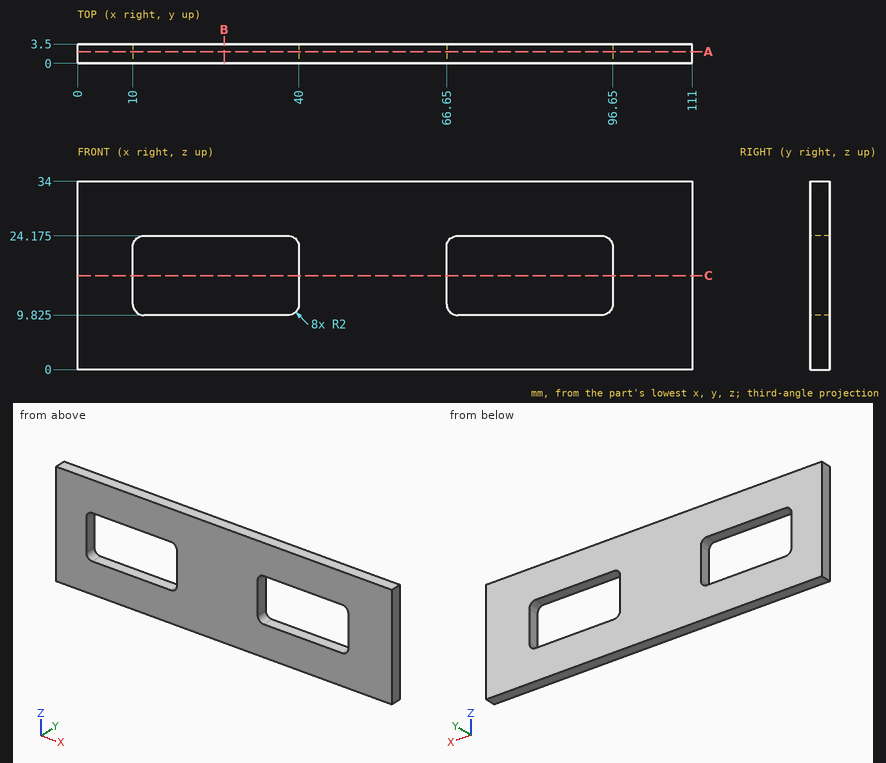
Design review of the part shown in the three views and the two pictorial views. Dimensions are in mm from the part's minimum x, y and z. Coordinates: 2 decimals unless noted, no trailing zeros. Loops run counter-clockwise (first coordinate to the right, second up) from the corner with the lowest first, then second, coordinate; pieces in that order, holes last. Notation, with made-up numbers: M 88,-29.5 L 105,-29.5 A30 cw 105,2.5 Z; hole C -25.75,26.5 d9. An arc over 180 degrees is marked long. Put each result on its own line as item: value. Start each with the question number.
Q1. Wall thickness on line 1 (X direction, y = 1.35, z = 13.5); line 2 (Z direction, x = 91, y = 1.4) (3 decimals); line 3 (X direction, y = 2.55, z = 10.5): over which ranges is each line inside the solid? List them lowest first.
Q2. Clearance check with a flat-ended pin moving along its axis: pin 1 (8 mm diameter, centred on x = 67, z = 23.5, fed in from -Y). State where the tip first meets the part, or that it passes through.
Q3. Add section C-C (z = 17). Write out the cut boundary in (x, y), and give its area (4 significant figures).
Q4. Add section B-B (x = 26.5). Write out the cut boundary in (y, z) (3 decimals).
Q5. Add section A-A (y = 2.1). Write out the cut boundary in (x, z) (3 decimals), and give its area (3 significant figures).
Answers:
1. line 1: x = 0 to 10, 40 to 66.65, 96.65 to 111
1. line 2: z = 0 to 9.825, 24.175 to 34
1. line 3: x = 0 to 10.5, 39.5 to 67.15, 96.15 to 111
2. pin 1: stops at y = 0
3. outline: M 0,0 L 10,0 L 10,3.5 L 0,3.5 Z; M 40,0 L 66.65,0 L 66.65,3.5 L 40,3.5 Z; M 96.65,0 L 111,0 L 111,3.5 L 96.65,3.5 Z
3. area: 178.5 mm^2
4. outline: M 0,0 L 3.5,0 L 3.5,9.825 L 0,9.825 Z; M 0,24.175 L 3.5,24.175 L 3.5,34 L 0,34 Z
5. outline: M 0,0 L 111,0 L 111,34 L 0,34 Z; hole M 10,11.825 A2 ccw 12,9.825 L 38,9.825 A2 ccw 40,11.825 L 40,22.175 A2 ccw 38,24.175 L 12,24.175 A2 ccw 10,22.175 Z; hole M 66.65,11.825 A2 ccw 68.65,9.825 L 94.65,9.825 A2 ccw 96.65,11.825 L 96.65,22.175 A2 ccw 94.65,24.175 L 68.65,24.175 A2 ccw 66.65,22.175 Z
5. area: 2,920 mm^2
